The model under review builds one solid part; all positions refer to its coordinate system, in mm. A direction names the side the tool comes from. Give positions to 0.01 mm unless a question says otherwise; leave off trailing zeros. Loops run counter-clockwise (first coordinate to the right, second up) from the corner with the lowest first, then second, coordinate; pieces in that order, holes last. Notation, with made-up numbers: (7, -27) - (26, -27) arc R19 ccw to (26, -1) - close; hole circle Ø5 at (15.25, 68.5). An arc over 180 degrees is marked (long way). Answer as a JSON object with one key per item and string values.
from build123d import *

# Parameters (mm, degrees)
SKETCH1_R           = 18
BASEKEY_DEPTH       = 25
RECTANGLE_DEPTH     = 25
RECTANGLEPAT_COUNT  = 8
SKETCH_1_R          = 10
CUT_EXTRUDE_1_DEPTH = 22
CUT_EXTRUDE_2_DEPTH = 14


with BuildPart() as part:
    # Sketch1 → BaseKey (new, symmetric)
    with BuildSketch(Plane.XY):
        Circle(SKETCH1_R)
    extrude(amount=BASEKEY_DEPTH, both=True)

    # Sketch2 → Rectangle (add, symmetric)
    with BuildSketch(Plane.XY):
        with BuildLine():
            Line((-3.5, 19.691368668), (-3.5, 0))
            Line((-3.5, 0), (3.5, 0))
            Line((3.5, 0), (3.5, 19.691368668))
            ThreePointArc((3.5, 19.691368668), (0, 20), (-3.5, 19.691368668))
        make_face()
    rectangle = extrude(amount=RECTANGLE_DEPTH, both=True)

    # RectanglePat: Rectangle ×8 about axis
    rectanglepat_axis = Axis((0, 0, 0), (0, 0, 1))
    for i in range(1, RECTANGLEPAT_COUNT):
        add(rectangle.rotate(rectanglepat_axis, i * 360 / RECTANGLEPAT_COUNT))

    # 草图1 → 切除-拉伸1 (cut)
    with BuildSketch(Plane(origin=(0, 0, -25), x_dir=(-1, 0, 0), z_dir=(0, 0, -1))):
        Circle(SKETCH_1_R)
    extrude(amount=-CUT_EXTRUDE_1_DEPTH, mode=Mode.SUBTRACT)

    # 草图3 → 切除-拉伸2 (cut)
    with BuildSketch(Plane(origin=(0, 0, 0), x_dir=(1, 0, 0), z_dir=(0, 1, 0))):
        Polygon((5, 25), (-5, 25), (-5, 18), (-5, 3), (5, 3), (5, 18), align=None)
    extrude(amount=CUT_EXTRUDE_2_DEPTH, mode=Mode.SUBTRACT)


solid = part.part
Q1. Consider section A-A, the plane y = 0. State the section outline as (x, z) points, plus the area to 3 significant figures.
Results:
{"outline": "(-20, -25) - (-10, -25) - (-10, -3) - (10, -3) - (10, -25) - (20, -25) - (20, 25) - (-20, 25) - close", "area": "1,560 mm^2"}
Q2. Clearance check with flat-ended pins moving along their axes: pin 1 Ø3 at (x, z) = (10.5, -10) entering from -Y; pin 2 Ø1.6 at (x, z) = (19, 8) entering from -Y; pin 3 Ø12 at (y, z) = (-8, 16.5) entering from -X. State where each tip first meets the part, or that it passes through.
Results:
{"pin 1": "stops at y = -16.4", "pin 2": "stops at y = -3.5", "pin 3": "stops at x = -19.9"}
Q3. For faces 1 (the face through (-19, -3.5, 0)), 2 (the face through (-16.611, 6.934, 0.35)), 3 (the face through (-5, 11, -14)), 4 (the face through (-19, 3.5, 0)), 5 (the face through (15.69, -10.74, 0.35)), list the 3-axis set-ups (+Z, -Z, +X, -X, +Y, -Y) from which the entire face can be reached by the end or side of a thin tool; tool diameter is ignored.
Results:
{"face 1": "+Z, -Z, -X, -Y", "face 2": "+Z, -Z, -X", "face 3": "-Z", "face 4": "+Z, -Z, -X, +Y", "face 5": "+Z, -Z, +X"}
Q4. The part is to be moulded in two halves that separate along Y. For faces 6 (the face through (6.934, 16.611, 0.35)), 7 (the face through (5, 11, -14)), 8 (the face through (-3.5, 19, 0)), say which applies: +Y half, -Y half, draft (parallel to the pull), parting line (faces both ways), or undercut.
Results:
{"face 6": "+Y half", "face 7": "undercut", "face 8": "draft"}
Q5. Consider section C-C, the plane x = 0. State the section outline as (y, z) points, plus the area to 3 significant figures.
Results:
{"outline": "(-20, -25) - (-10, -25) - (-10, -3) - (14, -3) - (14, -25) - (20, -25) - (20, 25) - (-20, 25) - close", "area": "1,470 mm^2"}
Q6. To check wall thickness, follow probe 1 along Y at (x, z) = (0, -14); probe 2 along Z at (x, y) = (-6, 5); probe 3 along X at (y, z) = (10, 2.5). State the ranges of each line that lie inside material, in increasing order. Write a range as [from, to].
Results:
{"probe 1": "y = [-20, -10], [14, 20]", "probe 2": "z = [-3, 25]", "probe 3": "x = [-14.97, 14.97]"}
